Autodesk Inventor part; units mm, degrees
ref_plane "YZ Plane" through (0, 0, 0) normal (1, 0, 0) x (0, 1, 0)
ref_plane "XZ Plane" through (0, 0, 0) normal (0, 1, 0) x (-1, 0, 0)
ref_plane "XY Plane" through (0, 0, 0) normal (0, 0, 1) x (1, 0, 0)
sketch "Esboço1" plane through (0, 0, 0) normal (1, 0, 0) x (0, 1, 0)
  line L0 (0, 0) -> (149.6, 0)
  line L1 (149.6, 0) -> (149.6, -71.5)
  line L2 (149.6, -71.5) -> (0, -71.5)
  line L3 (0, -71.5) -> (0, 0)
  dimension "d0" = 149.6
  dimension "d1" = 71.5
extrude "Extrusão1" add sketch "Esboço1" along normal blind 7.95
fillet "Arredondamento1" radius 13 4 edges at (3.975, 149.6, -71.5) (3.975, 149.6, 0) (3.975, 0, 0) (3.975, 0, -71.5)
fillet "Arredondamento2" radius 1 8 edges at (7.95, 0, -35.75) (7.95, 3.8076, -67.6924) (7.95, 74.8, -71.5) (7.95, 145.7924, -67.6924) (7.95, 149.6, -35.75) (7.95, 145.7924, -3.8076) (7.95, 74.8, 0) (7.95, 3.8076, -3.8076)
sketch "Esboço2" plane through (0, 0, -58.5) normal (0, -1, 0) x (1, 0, 0)
  line L0 (6.95, 0) -> (0, 0)
  line L1 (0, 45.5) -> (6.95, 45.5)
  line L2 (3.475, 18.65) -> (4.775, 18.65)
  line L3 (4.775, 18.65) -> (2.175, 18.65)
  line L4 (2.175, 18.65) -> (2.175, 26.85)
  line L5 (2.175, 26.85) -> (4.775, 26.85)
  line L6 (4.775, 26.85) -> (4.775, 18.65)
  point P0 (0, 58.5)
extrude "Extrusão2" cut sketch "Esboço2" against normal blind 6.2
fillet "Arredondamento3" radius 1.3 4 edges at (4.775, 3.1, -39.85) (2.175, 3.1, -39.85) (4.775, 3.1, -31.65) (2.175, 3.1, -31.65)
sketch "Esboço3" plane through (0, 6.2, -58.5) normal (0, -1, 0) x (1, 0, 0)
  arc A0 (4.775, 25.55) -> (2.175, 25.55) centre (3.475, 25.55) ccw
  arc A1 (2.175, 19.95) -> (4.775, 19.95) centre (3.475, 19.95) ccw
  line L0 (3.475, 25.55) -> (3.475, 19.95) construction
  line L1 (3.125, 25.55) -> (3.125, 19.95)
  line L2 (3.825, 19.95) -> (3.825, 25.55)
  arc A2 (3.825, 25.55) -> (3.125, 25.55) centre (3.475, 25.55) ccw
  arc A3 (3.125, 19.95) -> (3.825, 19.95) centre (3.475, 19.95) ccw
  point P0 (0, 58.5)
  point P1 (3.475, 22.75)
extrude "Extrusão3" add sketch "Esboço3" along normal blind 5.5
sketch "Esboço4" plane through (0, 0, 0) normal (-1, 0, 0) x (0, 0, 1)
  line L0 (-58.5, 149.6) -> (-13, 149.6)
  arc A0 (-58.5, 148.6) -> (-70.5, 136.6) centre (-58.5, 136.6) ccw
  line L1 (-66.5, 131.06) -> (-66.5, 110.31)
  line L2 (-45, 110.31) -> (-45, 131.06)
  arc A1 (-45, 131.06) -> (-66.5, 131.06) centre (-55.75, 131.06) ccw
  arc A2 (-66.5, 110.31) -> (-45, 110.31) centre (-55.75, 110.31) ccw
  circle A3 centre (-55.75, 131.06) radius 8.4
  circle A4 centre (-55.75, 131.06) radius 7.6
  circle A5 centre (-55.75, 131.06) radius 5.75
  circle A6 centre (-55.75, 110.31) radius 8.4
  circle A7 centre (-55.75, 110.31) radius 7.6
  circle A8 centre (-55.75, 110.31) radius 5.75
  point P0 (0, 0)
extrude "Extrusão4" add sketch "Esboço4" along normal blind 2.2 contours A1 L2 A2 L1
sketch "Esboço5" plane through (0, 0, 0) normal (-1, 0, 0) x (0, 0, 1)
  circle A0 centre (-55.75, 131.06) radius 8.4
  circle A1 centre (-55.75, 131.06) radius 7.6
  circle A2 centre (-55.75, 131.06) radius 5.75
  circle A3 centre (-55.75, 131.06) radius 8.4
  point P0 (0, 0)
extrude "Extrusão5" add sketch "Esboço5" along normal blind 3.3 contours A0
sketch "Esboço6" plane through (0, 131.06, -55.75) normal (-1, 0, 0) x (0, 0, 1)
  circle A0 centre (0, -20.75) radius 8.4
  circle A1 centre (0, -20.75) radius 8.4
  circle A2 centre (0, -20.75) radius 7.6
  point P0 (55.75, -131.06)
extrude "Extrusão6" add sketch "Esboço6" along normal blind 3.3
sketch "Esboço7" plane through (0, 131.06, -55.75) normal (-1, 0, 0) x (0, 0, 1)
  circle A0 centre (0, 0) radius 7.6
  circle A1 centre (0, -20.75) radius 7.6
  circle A2 centre (0, -20.75) radius 7.6
  point P0 (55.75, -131.06)
  dimension "d38" = 15.2
  dimension "d40" = 15.2
extrude "Extrusão7" add sketch "Esboço7" along normal blind 3.1
sketch "Esboço8" plane through (0, 0, 0) normal (-1, 0, 0) x (0, 0, 1)
  line L0 (-45, 110.31) -> (-45, 131.06)
  circle A0 centre (-35.7, 120.685) radius 2.5
  circle A1 centre (-35.7, 120.685) radius 2.3
  point P0 (0, 0)
  dimension "d45" = 4.6
extrude "Extrusão8" add sketch "Esboço8" along normal blind 0.2 contours A0 | A1
sketch "Esboço9" plane through (0, 13, 0) normal (0, 0, 1) x (1, 0, 0)
  line L0 (0, 136.6) -> (6.95, 136.6)
  line L1 (2.375, 103) -> (2.375, 97.2)
  line L2 (4.575, 97.2) -> (4.575, 103)
  arc A0 (4.575, 103) -> (2.375, 103) centre (3.475, 103) ccw
  arc A1 (2.375, 97.2) -> (4.575, 97.2) centre (3.475, 97.2) ccw
  line L3 (3.475, 79.35) -> (3.475, 90.85) construction
  line L4 (4.575, 79.35) -> (4.575, 90.85)
  line L5 (2.375, 90.85) -> (2.375, 79.35)
  arc A2 (2.375, 79.35) -> (4.575, 79.35) centre (3.475, 79.35) ccw
  arc A3 (4.575, 90.85) -> (2.375, 90.85) centre (3.475, 90.85) ccw
  point P0 (0, -13)
sketch "Esboço10" plane through (0, 13, 0) normal (0, 0, 1) x (1, 0, 0)
  line L0 (3.4735, 64.3614) -> (3.4735, 75.8614) construction
  line L1 (4.5735, 64.3614) -> (4.5735, 75.8614)
  line L2 (2.3735, 75.8614) -> (2.3735, 64.3614)
  arc A0 (2.3735, 64.3614) -> (4.5735, 64.3614) centre (3.4735, 64.3614) ccw
  arc A1 (4.5735, 75.8614) -> (2.3735, 75.8614) centre (3.4735, 75.8614) ccw
  point P0 (0, -13)
extrude "Extrusão9" add sketch "Esboço9" along normal blind 0.6
The listing builds one solid part. Answer for the finished solid, in the listing's coordinates (mm). A direction names the side the tool comes from. Coordinates: 2 decimals unless noted, no trailing zeros. Order: outer loops, then holes, each group sorted by start corner. A loop starts at its lowest first (then second) coordinate and runs counter-clockwise, first axis right, second up.
Q1. Consider line 1 (Y direction, x = -3.2, z = -55.75); line 2 (Z direction, x = 1, y = 112.5); line 3 (X direction, y = 53.5, z = -62). Determine where each line is inside the solid, lowest interval first.
Q2. Which of the six approach directions +Z, -Z, +X, -X, +Y, -Y give full straight-line access (tool end or side, diameter ignored) to faces 4 (the face through (-1.085, 99.563, -55.514)), 5 (the face through (7.95, 74, -35)), 6 (the face through (4.775, 3, -36)), 7 (the face through (-3.1, 131, -56)), 8 (the face through (-1.085, 141.807, -55.986))?
Q3. For a pull along X with two mould halves and no side action, classify faces 1 (the face through (3.524, 145.691, -67.793)), 2 (the face through (-3.1, 110, -56)), 3 (the face through (2.9, 6.2, -35.7)) as pulls with the +X half, pulls with the -X half, needs draft (parallel to the pull), parting line crosses it, or undercut.
Q4. Given P1, Ø1.8, axis at x = -1.5, y = 115.5, coming from the +Z side; P2, Ø0.7, axis at y = 96.5, z = 0.5, coming from the +X side (3 decimals); P3, Ø0.5, axis at y = 112.5, z = 0, coming from the +X side, each flat-ended and moving along its own axis, determine where each tip first touches the part or whether it passes through.
Q5. A cutting plane is placed at B-B, the plane z = -35.7. Write down the section's boundary in (x, y) (3 decimals).
Q6. A cutting plane is placed at A-A, the plane y = 42. Write down the section's boundary in (x, z).
Answers follow:
1. line 1: y = 101.91 to 102.71, 117.91 to 118.71, 122.66 to 123.46, 138.66 to 139.46
1. line 2: z = -71.5 to 0
1. line 3: x = 0 to 7.95
2. face 4: -X, -Y
2. face 5: +Z, -Z, +X, +Y, -Y
2. face 6: -Y
2. face 7: -X
2. face 8: -X, +Y
3. face 1: needs draft
3. face 2: pulls with the -X half
3. face 3: undercut
4. P1: stops at z = -45
4. P2: stops at x = 4.575
4. P3: stops at x = 7.61
5. outline: (-0.2, 118.185) - (0, 118.185) - (0, 0) - (2.175, 0) - (2.175, 6.2) - (3.125, 6.2) - (3.125, 0.7) - (3.825, 0.7) - (3.825, 6.2) - (4.775, 6.2) - (4.775, 0) - (6.95, 0) arc R1 ccw to (7.95, 1) - (7.95, 148.6) arc R1 ccw to (6.95, 149.6) - (0, 149.6) - (0, 123.185) - (-0.2, 123.185) - close
6. outline: (0, -71.5) - (6.95, -71.5) arc R1 ccw to (7.95, -70.5) - (7.95, -1) arc R1 ccw to (6.95, 0) - (0, 0) - close
